Design review of the part built by this model. Coordinates are the model's own, in mm. A direction names the side the tool comes from. Round coordinates to 2 decimals unless told otherwise and drop trailing zeros. Write each loop counter-clockwise with the first axis right and the second up, starting at its lowest first coordinate (ties: lowest second). Pieces come first, ordered by that corner, then holes. Notation, with made-up numbers: (56.5, 76.5) - (101.5, 76.5) arc R29 cw to (101.5, 110.5) - close; hole circle Ø1 at (20.5, 34.5). An arc over 180 degrees is marked (long way). Use one line per item in the form item = value.
```python
from build123d import *

# Parameters (mm, degrees)
SKETCH1_R           = 3.2639
BOSS_EXTRUDE1_DEPTH = 6.35
SKETCH2_W           = 50.8
SKETCH2_H           = 6.5278
CUT_EXTRUDE1_DEPTH  = 633.86660682


with BuildPart() as part:
    # Sketch1 → Boss-Extrude1 (new body)
    with BuildSketch(Plane(origin=(0, 345.441352572, 10.725757471), x_dir=(1, 0, 0), z_dir=(0, 0.9995183146693659, 0.0310344750319807))):
        with BuildLine():
            Line((-170.726579561, 560.338454563), (-272.326579561, 560.338454563))
            ThreePointArc((-272.326579561, 560.338454563), (-278.738498836, 557.857098237), (-281.809681848, 551.705864791))
            Line((-281.809681848, 551.705864791), (-293.761055515, 424.705864791))
            ThreePointArc((-293.761055515, 424.705864791), (-288.089455083, 415.084303481), (-277.177301788, 417.464724444))
            Line((-277.177301788, 417.464724444), (-163.62592812, 544.464724444))
            ThreePointArc((-163.62592812, 544.464724444), (-162.031831739, 554.702797092), (-170.726579561, 560.338454563))
        make_face()
        with Locations(Location((-284.277953229, 423.813454563, 0), (0, 0, 270))):
            Circle(SKETCH1_R, mode=Mode.SUBTRACT)
        with Locations(Location((-272.326579561, 550.813454563, 0), (0, 0, 270))):
            Circle(SKETCH1_R, mode=Mode.SUBTRACT)
        with Locations(Location((-170.726579561, 550.813454563, 0), (0, 0, 270))):
            Circle(SKETCH1_R, mode=Mode.SUBTRACT)
    extrude(amount=BOSS_EXTRUDE1_DEPTH)

    # Sketch2 → Cut-Extrude1 (cut, through all)
    with BuildSketch(Plane(origin=(0, 351.78829387, 10.922826388), x_dir=(1, 0, 0), z_dir=(0, 0.9995183146693659, 0.03103447503198071))):
        with Locations((-221.526579561, 550.813454563)):
            Rectangle(SKETCH2_W, SKETCH2_H)
    extrude(amount=-CUT_EXTRUDE1_DEPTH, mode=Mode.SUBTRACT)


solid = part.part
```
Q1. Draft analysis for pull direction X (two halves, no side actions). For faces 3 (the cylindrical face through (-161.97, 365.78, -543.47)), 4 (the cylindrical face through (-288.24, 361.45, -404.13)), 5 (the flat face through (-196.127, 366, -540)), state which applies: released by +X, released by -X, zero draft, split by the parting line, or undercut.
Calculated:
face_3 = released by +X
face_4 = split by the parting line
face_5 = undercut
Q2. We need section D-D on z = -453. Write out the cut boundary in (x, y), then the cut area to 3 significant figures.
Calculated:
outline = (-290.07, 359.84) - (-235.62, 359.84) - (-235.44, 366.19) - (-290.05, 366.19) - close
area = 346 mm2
Q3. We need section C-C on x = -198.5. Write out the cut boundary in (y, z), then the cut area to 3 significant figures.
Calculated:
outline = (361.13, -494.49) - (362.43, -536.56) - (368.78, -536.36) - (367.47, -494.29) - close; (362.64, -543.08) - (362.83, -549.34) - (369.18, -549.15) - (368.98, -542.89) - close
area = 307 mm2
Q4. We need section A-A on x = -236. Write out the cut boundary in (y, z).
Calculated:
outline = (359.83, -452.57) - (362.43, -536.56) - (368.78, -536.36) - (366.17, -452.37) - close; (362.64, -543.08) - (362.83, -549.34) - (369.18, -549.15) - (368.98, -542.89) - close
Q5. For P1, Ø1, axis at y = 362, z = -527.5, coming from the -X side; P2, Ø4, axis at x = -242.5, y = 368, coming from the -Z side; P3, Ø4, axis at x = -262.5, z = -514, coming from the -Y side, all flat-tipped, find the tip position at first contact; note any pin that passes through.
Calculated:
P1 = -283.1
P2 = -549.24
P3 = 361.67
Q6. We need section B-B on z = -508.5. Write out the cut boundary in (x, y).
Calculated:
outline = (-284.84, 361.56) - (-185.97, 361.56) - (-185.79, 367.92) - (-284.82, 367.92) - close
Q7. Machinability: for faces 1 (the cylindrical face through (-173.913, 365.687, -540.432)), 2 (the cylindrical face through (-278.7, 365.9, -546.8)), which of the approach directions +Z, -Z, +X, -X, +Y, -Y give a long, thin tool a straight path to every point of the face, cutting with its end or side? Answer none if there is none.
Calculated:
face_1 = none
face_2 = -Z, -X, +Y
Q8. To check wall thickness, follow line 1 along X through (y, z) = (367.5, -540); line 2 along Y through (x, z) = (-218, -533); line 3 along Z through (x, y) = (-201.5, 366.5). State the ranges of each line that lie inside material, in increasing order. Write a range as from..to.
Calculated:
line_1 = -281.86..-275.57, -269.08..-246.93, -196.13..-173.97, -167.48..-161.21
line_2 = 362.32..368.68
line_3 = -549.23..-542.96, -536.43..-490.97
